Build history of the part. All positions in model axes, mm. Face numbers are marked on the shaded views. A direction names the side the tool comes from. Give positions to 0.01 mm unless a question says otherwise; leave off trailing zeros. Loops run counter-clockwise (first coordinate to the right, second up) from the corner with the lowest first, then second, coordinate; pieces in that order, holes last. Notation, with made-up numbers: M -11,46 L 20,46 A14 cw 20,68 Z; hole C -18.5,30 d10. An arc over 180 degrees is marked long. Answer as a JSON object with one key per item and string values. Group by question number.
1. Drop flat-ended pins along their axis: pin 1 Ø1 at (x, z) = (3, 1) entering from -Y; pin 2 Ø1 at (x, y) = (0, 12) entering from +Z; pin 3 Ø4 at (y, z) = (18.5, 4.5) entering from +X; pin 4 Ø2 at (x, y) = (3.5, 30) entering from +Z. Give the stop position or say it passes through.
2. Drill centre lines: line 1 along Y through (x, z) = (-3.75, 7); line 2 along X through (y, z) = (12.5, -5) (3 decimals); line 3 along X through (y, z) = (6, -2.5). Where is each one in solid material? Low to high. Write a range as [from, to].
3. Slice it at A-A (y = 9). List the corners of the cut face in (x, z).
4. 3-axis set-ups, long thin cutter, end or side, ignore diameter. For the marked faces 1 and 2: which of +Z, -Z, +X, -X, +Y, -Y reach the whole face in a straight line?
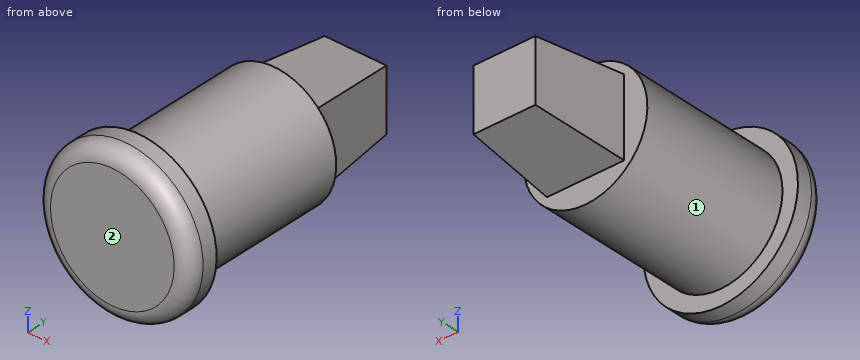
from build123d import *


with BuildPart() as part:
    # Sketch1 → Revolve1 (revolve)
    with BuildSketch(Plane.XY, mode=Mode.PRIVATE) as revolve1_sk:
        with BuildLine():
            Line((0, 0), (0, 24))
            Line((0, 24), (8, 24))
            Line((8, 24), (8, 4))
            Line((8, 4), (10, 4))
            Line((10, 4), (10, 2))
            ThreePointArc((10, 2), (9.414213562, 0.585786438), (8, 0))
            Line((8, 0), (0, 0))
        make_face()
    revolve(revolve1_sk.sketch.rotate(Axis((0, 0, 0), (0, 1, 0)), 90), axis=Axis((0, 0, 0), (0, 1, 0)))

    # Sketch3 → Loft1 section 0
    with BuildSketch(Plane(origin=(0, 36, 0), x_dir=(1, 0, 0), z_dir=(0, 1, 0))):
        with BuildLine():
            Line((-4, -4), (4, -4))
            Line((4, -4), (4, 4))
            Line((4, 4), (-4, 4))
            Line((-4, 4), (-4, -4))
        make_face()
    # Sketch2 → Loft1 section 1
    with BuildSketch(Plane(origin=(0, 24, 0), x_dir=(1, 0, 0), z_dir=(0, 1, 0))):
        with BuildLine():
            Line((-5, -5), (5, -5))
            Line((5, -5), (5, 5))
            Line((5, 5), (-5, 5))
            Line((-5, 5), (-5, -5))
        make_face()
    loft()


solid = part.part
Established:
{
 "1": {"pin 1": "stops at y = 0", "pin 2": "stops at z = 8", "pin 3": "stops at x = 7.6", "pin 4": "stops at z = 4.58"},
 "2": {"line 1": "y = [0, 24]", "line 2": "x = [-6.245, 6.245]", "line 3": "x = [-7.6, 7.6]"},
 "3": {"outline": "C 0,0 d16"},
 "4": {"face 1": "+Y", "face 2": "+Z, -Z, +X, -X, -Y"}
}
